```python
from build123d import *

# Parameters (mm, degrees)
F0_R     = 1.5
F0_W     = 22.86
F0_H     = 25.4
F1_DEPTH = 3.175


# Not quite as in the source:
# - a length typed as a fraction of an inch, garbled in the dataset ("3 / 203.2 mm" for 3/8 in), is restored


with BuildPart() as f1:
    # F0 (on Top) → F1 (new body)
    with BuildSketch(Plane.XY):
        Polygon((-41.8889727067, -63.5), (-24.765, -63.5), (-24.765, -60.325), (-17.907, -60.325), (-17.907, -57.785), (-19.939, -57.785), (-19.939, -55.245), (-17.907, -55.245), (-17.907, -52.705), (-15.113, -52.705), (-15.113, -55.245), (-13.081, -55.245), (-13.081, -57.785), (-15.113, -57.785), (-15.113, -60.325), (-8.255, -60.325), (-8.255, -63.5), (8.255, -63.5), (8.255, -60.325), (15.113, -60.325), (15.113, -57.785), (13.081, -57.785), (13.081, -55.245), (15.113, -55.245), (15.113, -52.705), (17.907, -52.705), (17.907, -55.245), (19.939, -55.245), (19.939, -57.785), (17.907, -57.785), (17.907, -60.325), (24.765, -60.325), (24.765, -63.5), (41.8889727067, -63.5), (41.91, -63.5), (45.0639727067, -63.5), (45.0639727067, -38.1), (41.8889727067, -38.1), (41.8889727067, -12.7), (45.0639727067, -12.7), (45.0639727067, 12.7), (41.8889727067, 12.7), (41.8889727067, 38.1), (24.765, 38.1), (24.765, 34.925), (17.907, 34.925), (17.907, 32.385), (19.939, 32.385), (19.939, 29.845), (17.907, 29.845), (17.907, 27.305), (15.113, 27.305), (15.113, 29.845), (13.081, 29.845), (13.081, 32.385), (15.113, 32.385), (15.113, 34.925), (8.255, 34.925), (8.255, 38.1), (-8.255, 38.1), (-8.255, 34.925), (-15.113, 34.925), (-15.113, 32.385), (-13.081, 32.385), (-13.081, 29.845), (-15.113, 29.845), (-15.113, 27.305), (-17.907, 27.305), (-17.907, 29.845), (-19.939, 29.845), (-19.939, 32.385), (-17.907, 32.385), (-17.907, 34.925), (-24.765, 34.925), (-24.765, 38.1), (-41.8889727067, 38.1), (-41.8889727067, 12.7), (-45.0639727067, 12.7), (-45.0639727067, -12.7), (-41.8889727067, -12.7), (-41.8889727067, -38.1), (-45.0639727067, -38.1), (-45.0639727067, -63.5), (-41.91, -63.5), align=None)
        with Locations((-43.4764727067, -50.8)):
            Circle(F0_R, mode=Mode.SUBTRACT)
        with Locations((43.4764727067, -50.8)):
            Circle(F0_R, mode=Mode.SUBTRACT)
        with Locations((-43.4764727067, 0)):
            Circle(F0_R, mode=Mode.SUBTRACT)
        with Locations((-14.4632559413, 8.0235061839)):
            Rectangle(F0_W, F0_H, mode=Mode.SUBTRACT)
        with Locations((14.4632559413, 8.2762846043)):
            Rectangle(F0_W, F0_H, mode=Mode.SUBTRACT)
        with Locations((43.4764727067, 0)):
            Circle(F0_R, mode=Mode.SUBTRACT)
    extrude(amount=F1_DEPTH)


solid = f1.part
```
Check sheet for the modelled part. Datum: model origin and axes. Units: mm. A direction names the side the tool comes from. Round coordinates to 2 decimals unless told otherwise and drop trailing zeros. Order: outer loops, then holes, each group sorted by start corner. A loop starts at its lowest first (then second) coordinate and runs counter-clockwise, first axis right, second up. Notation, with made-up numbers: (2, 40) -> (36, 40) arc R10 cw to (36, 55) -> close; hole circle Ø6 at (56.25, 80). An arc over 180 degrees is marked (long way). One line per item, written item: value. Start each with the question number.
Q1. Cross-section at A-A (y = 0). Record the boundary of the cut face in (x, z) (3 decimals).
Q2. Cross-section at C-C (z = 2.1). Give the number of separate pieces and of enclosed holes in the cut face, and give its area (3 significant figures).
Q3. Gauge pin test, flat ends, axial feed: pin 1 Ø1 at (x, z) = (10, 2.5) entering from -Y (3 decimals); pin 2 Ø1 at (y, z) = (-30.5, 1.5) entering from +X; pin 3 Ø1 at (x, z) = (19.5, 1) entering from +Y (3 decimals). Record the tip position at first contact, or that the pin passes through.
Q4. Set-up check for faces 5 (the face through (43, -38.1, 2)), 6 (the face through (-15.113, 34, 2)), 7 (the face through (8.255, -62, 2)): record each of +Z, -Z, +X, -X, +Y, -Y from which the full face is reachable in a straight line by a thin tool's end or side.
Q5. Mould release check, pull along Y, two halves, no side actions. Record for faces 1 (the face through (16, -52.705, 2)), 2 (the face through (-15, 20.724, 2)), 3 (the face through (14, 20.976, 2)), 4 (the face through (24.765, -62, 2)): pulls with the +Y half, pulls with the -Y half, needs draft (parallel to the pull), parting line crosses it, or undercut.
Q6. Cross-section at B-B (y = 16.5). Record the boundary of the cut face in (x, z) (3 decimals), and give its area (3 significant figures).
Q7. Cross-section at D-D (y = -50.8). Record the boundary of the cut face in (x, z) (3 decimals), and give its area (3 significant figures).
Q8. Thickness scan on line 1 (X direction, y = -54.5, z = 2.7); line 2 (Y direction, x = 24.5, z = 2.2) (3 decimals); line 3 (X direction, y = 3.5, z = 3.05). Record the ranges inside material, lowest first.
Completed:
1. outline: (-45.064, 0) -> (-44.976, 0) -> (-44.976, 3.175) -> (-45.064, 3.175) -> close; (-41.976, 0) -> (-25.893, 0) -> (-25.893, 3.175) -> (-41.976, 3.175) -> close; (-3.033, 0) -> (3.033, 0) -> (3.033, 3.175) -> (-3.033, 3.175) -> close; (25.893, 0) -> (41.976, 0) -> (41.976, 3.175) -> (25.893, 3.175) -> close; (44.976, 0) -> (45.064, 0) -> (45.064, 3.175) -> (44.976, 3.175) -> close
2. separate pieces: 1
2. enclosed holes: 6
2. area: 7,310 mm²
3. pin 1: stops at y = -60.325
3. pin 2: stops at x = 41.89
3. pin 3: stops at y = 34.925
4. face 5: +Z, -Z, +X
4. face 6: +Z, -Z, +Y
4. face 7: +Z, -Z, -Y
5. face 1: pulls with the -Y half
5. face 2: undercut
5. face 3: undercut
5. face 4: needs draft
6. outline: (-41.889, 0) -> (-25.893, 0) -> (-25.893, 3.175) -> (-41.889, 3.175) -> close; (-3.033, 0) -> (3.033, 0) -> (3.033, 3.175) -> (-3.033, 3.175) -> close; (25.893, 0) -> (41.889, 0) -> (41.889, 3.175) -> (25.893, 3.175) -> close
6. area: 121 mm²
7. outline: (-45.064, 0) -> (-44.976, 0) -> (-44.976, 3.175) -> (-45.064, 3.175) -> close; (-41.976, 0) -> (41.976, 0) -> (41.976, 3.175) -> (-41.976, 3.175) -> close; (44.976, 0) -> (45.064, 0) -> (45.064, 3.175) -> (44.976, 3.175) -> close
7. area: 267 mm²
8. line 1: x = -45.06 to -17.91, -15.11 to 15.11, 17.91 to 45.06
8. line 2: y = -60.325 to -4.424, 20.976 to 34.925
8. line 3: x = -45.06 to -25.89, -3.03 to 3.03, 25.89 to 45.06
